Answer from the drawing. Dimensions are ordinates in mm from the lowest x, y and z of the part. A direction names the side the tool comes from. Give positions to 0.01 mm unless a question says otherwise; leave off trailing zeros. Write each loop counter-clockwise with the first axis right and the second up, starting at its lowest first coordinate (ties: lowest second). Pieces come first, ordered by that corner, then holes. Notation, with made-up numbers: (-7, 12) -> (33, 12) arc R26 cw to (33, 43) -> close; hole circle Ø3 at (-36.75, 21.5). An arc over 180 degrees is marked (long way). Use a Markdown table: item, result. Add a question column.
Q1. Consider line 1 (Y direction, x = 14, z = 2.2); line 2 (X direction, y = 15, z = 2); line 3 (Z direction, x = 5.5, y = 8.5). Determine where each line is inside the solid, lowest interval first.
Q2. Section C-C, the plane z = 5 is taken. Give the vertices of the cut face in (x, y), plus the area to 3 significant figures.
Q3. Each of these flat-tipped pins is pushed along its axis until it touches: pin 1 Ø2 at (x, y) = (20.5, 23) entering from +Z; pin 2 Ø6.5 at (x, y) = (14, 14) entering from +Z; pin 3 Ø2 at (x, y) = (4.5, 20) entering from -Z. Where does it stop, or does it pass through?
Q4. Section B-B, the plane z = 0.5 is taken. Give the vertices of the cut face in (x, y).
Q5. For a pull along X with two mould halves and no side action, classify the marked faces 3, 4 and 5 as pulls with the +X half, pulls with the -X half, needs draft (parallel to the pull), parting line crosses it, or undercut.
Q6. Section A-A, the plane x = 14 is taken. Give the vertices of the cut face in (y, z).
Q7. For the marked faces 1 and 2, determine the directions among +Z, -Z, +X, -X, +Y, -Y from which every point of the face is accessible in a straight line to the end or side of a thin tool.
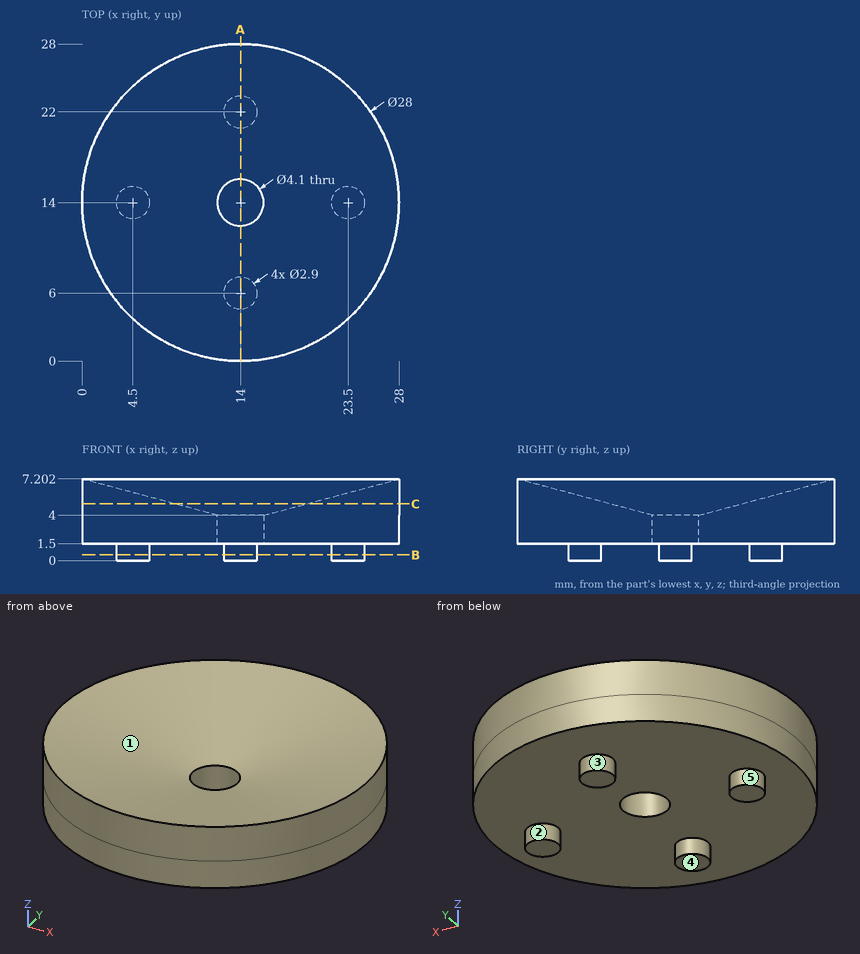
Result set:
| question | item | result |
|---|---|---|
| 1 | line 1 | y = 0 to 11.95, 16.05 to 28 |
| 1 | line 2 | x = 0.04 to 12.21, 15.79 to 27.96 |
| 1 | line 3 | z = 1.5 to 6.16 |
| 2 | outline | circle Ø28 at (14, 14); hole circle Ø11.56 at (14, 14) |
| 2 | area | 511 mm2 |
| 3 | pin 1 | stops at z = 6.69 |
| 3 | pin 2 | stops at z = 4.32 |
| 3 | pin 3 | stops at z = 1.5 |
| 4 | outline | circle Ø2.9 at (4.5, 14); circle Ø2.9 at (14, 6); circle Ø2.9 at (14, 22); circle Ø2.9 at (23.5, 14) |
| 5 | face 3 | parting line crosses it |
| 5 | face 4 | needs draft |
| 5 | face 5 | undercut |
| 6 | outline | (0, 1.5) -> (4.55, 1.5) -> (4.55, 0) -> (7.45, 0) -> (7.45, 1.5) -> (11.95, 1.5) -> (11.95, 4) -> (0, 7.2) -> close; (16.05, 1.5) -> (20.55, 1.5) -> (20.55, 0) -> (23.45, 0) -> (23.45, 1.5) -> (28, 1.5) -> (28, 7.2) -> (16.05, 4) -> close |
| 7 | face 1 | +Z |
| 7 | face 2 | -Z |
